from build123d import *

# Parameters (mm, degrees)
F0_R     = 30
F1_DEPTH = 35
F0_R_2   = 45
F2_DEPTH = 25
F3_R     = 19.112105
F4_DEPTH = 45


with BuildPart() as f1:
    # F0 (on Front) → F1 (new body, symmetric)
    with BuildSketch(Plane.XZ):
        Circle(F0_R)
    extrude(amount=F1_DEPTH, both=True)

    # F0 (on Front) → F2 (join, symmetric)
    with BuildSketch(Plane.XZ):
        Circle(F0_R_2)
        Circle(F0_R, mode=Mode.SUBTRACT)
    extrude(amount=F2_DEPTH, both=True)

    # F3 (on Right) → F4 (cut, symmetric)
    with BuildSketch(Plane.YZ):
        Circle(F3_R)
    extrude(amount=F4_DEPTH, both=True, mode=Mode.SUBTRACT)


solid = f1.part
Geometry: final body of the model. Coordinates: model frame, mm. A direction names the side the tool comes from. Give positions to 0.01 mm unless a question says otherwise; leave off trailing zeros. Loops run counter-clockwise (first coordinate to the right, second up) from the corner with the lowest first, then second, coordinate; pieces in that order, holes last. Notation, with made-up numbers: (-11.75, 80.5) -> (39.25, 80.5) arc R25 cw to (39.25, 94.5) -> close; hole circle Ø11 at (69, 53.5). An arc over 180 degrees is marked (long way). Put each result on its own line as item: value.
1. Cut plane A-A (z = 0). Return the cut outline in (x, y).
Taken from the geometry:
outline: (-45, -25) -> (-30, -25) -> (-30, -35) -> (30, -35) -> (30, -25) -> (45, -25) -> (45, -19.11) -> (-45, -19.11) -> close; (-45, 19.11) -> (45, 19.11) -> (45, 25) -> (30, 25) -> (30, 35) -> (-30, 35) -> (-30, 25) -> (-45, 25) -> close
2. Cut plane B-B (x = 0). Return the cut outline in (y, z).
Taken from the geometry:
outline: (-35, -30) -> (-25, -30) -> (-25, -45) -> (25, -45) -> (25, -30) -> (35, -30) -> (35, 30) -> (25, 30) -> (25, 45) -> (-25, 45) -> (-25, 30) -> (-35, 30) -> close; hole circle Ø38.22 at (0, 0)
3. Cut plane D-D (z = -25.5). Return the cut outline in (x, y), plus the area to 3 significant figures.
Taken from the geometry:
outline: (-37.08, -25) -> (-15.8, -25) -> (-15.8, -35) -> (15.8, -35) -> (15.8, -25) -> (37.08, -25) -> (37.08, 25) -> (15.8, 25) -> (15.8, 35) -> (-15.8, 35) -> (-15.8, 25) -> (-37.08, 25) -> close
area: 4,340 mm2
4. Ray query, line 1 along Y through (x, z) = (-22, 0); line 2 along Z through (x, y) = (-1, 0); line 3 along Z through (x, y) = (3, 0). Return the intervals inside material, ascending. Write a range as [from, to].
Taken from the geometry:
line 1: y = [-35, -19.11], [19.11, 35]
line 2: z = [-44.99, -19.11], [19.11, 44.99]
line 3: z = [-44.9, -19.11], [19.11, 44.9]
5. Pull-direction query (Y, two-part tool) for faces 1 (the flat face through (0, -35, 0)), 2 (the cylindrical face through (-29.97, -30.07, 1.32)), 3 (the flat face through (29, 25, -9)), 4 (the cylindrical face through (0.629, -15.167, -11.629)); classes: released by +Y, released by -Y, zero draft, split by the parting line, or undercut.
Taken from the geometry:
face 1: released by -Y
face 2: zero draft
face 3: released by +Y
face 4: undercut
6. Pin query (flat end, axial travel): P1, Ø4, axis at y = 25.5, z = 24, coming from the +X side; P2, Ø4, axis at y = -21, z = -14.5, coming from the -X side; P3, Ø10, axis at x = 35.5, y = 4, coming from the +Z side. Return the tip coordinate at first contact, or that it passes through.
Taken from the geometry:
P1: stops at x = 39.22
P2: stops at x = -43.23
P3: stops at z = 33.09
7. Set-up query: faces 5 (the flat face through (0, 35, 0)), 6 (the cylindrical face through (-29.97, 29.93, 1.32)), 7 (the flat face through (29, -25, -9)). Return all of +Z, -Z, +X, -X, +Y, -Y with unobstructed straight access to the full face (end or side cutting, diameter ignored); none if empty.
Taken from the geometry:
face 5: +Z, -Z, +X, -X, +Y
face 6: +Y
face 7: -Y
8. Cut plane C-C (y = 3.5). Return the cut outline in (x, z), plus the area to 3 significant figures.
Taken from the geometry:
outline: (-40.89, -18.79) arc R45 ccw to (40.89, -18.79) -> close; (-40.89, 18.79) -> (40.89, 18.79) arc R45 ccw to start
area: 3,080 mm2
